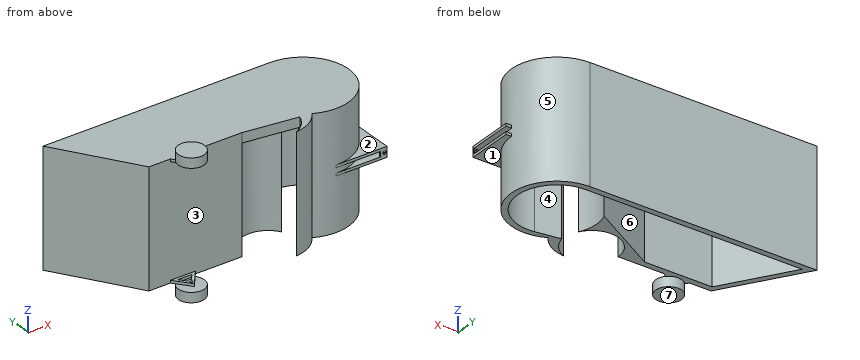
```python
from build123d import *

# Parameters (mm, degrees)
BOSS_EXTRUDE1_DEPTH = 897
SKETCH2_R           = 10.767041916
BOSS_EXTRUDE2_DEPTH = 20
BOSS_EXTRUDE3_START = 20
BOSS_EXTRUDE3_DEPTH = 20
SKETCH4_W           = 50
SKETCH4_H           = 50
SKETCH4_R           = 12.5
BOSS_EXTRUDE4_DEPTH = 10
SKETCH5_R           = 100
BOSS_EXTRUDE5_DEPTH = 75
BOSS_EXTRUDE6_START = -75
BOSS_EXTRUDE6_DEPTH = 75


with BuildPart() as part:
    # Sketch1 → Boss-Extrude1 (new body)
    with BuildSketch(Plane.XY):
        with BuildLine():
            add(Edge.make_bspline(
                [(80.115553735, -191.384207833), (181.903017437, -142.41499007), (210.702960853, -28.558773965)],
                knots=[0, 0, 0, 1, 1, 1], degree=2))
            Line((210.702960853, -28.558773965), (401.206683232, -56.895630445))
            ThreePointArc((401.206683232, -56.895630445), (750.24986995, 222.286833017), (446.080798211, 549.785184001))
            Line((446.080798211, 549.785184001), (-1220.08310634, 549.785184001))
            Line((-1220.08310634, 549.785184001), (-894.475187417, 45))
            Line((-894.475187417, 45), (-374.993230006, 45))
            Line((-374.993230006, 45), (160.769466444, 352.592623287))
            ThreePointArc((160.769466444, 352.592623287), (141.659115875, 226.01181659), (176.177724746, 102.738251846))
            ThreePointArc((176.177724746, 102.738251846), (-53.212296367, 196.881158582), (-203.945431646, 0))
            Line((-203.945431646, 0), (-918.997892597, 0))
            Line((-918.997892597, 0), (-1302.659640419, 594.785184001))
            Line((-1302.659640419, 594.785184001), (446.080798211, 594.785184001))
            ThreePointArc((446.080798211, 594.785184001), (786.541848074, 163.629324532), (288.192746113, -67.578967279))
            add(Edge.make_bspline(
                [(80.115553735, -191.384207833), (212.051449387, -178.806537551), (288.192746113, -67.578967279)],
                knots=[0, 0, 0, 1, 1, 1], degree=2))
        make_face()
    extrude(amount=BOSS_EXTRUDE1_DEPTH)

    # Sketch2 → Boss-Extrude2 (add)
    with BuildSketch(Plane.XY.offset(897)):
        Polygon((-753.618518266, 0), (-561.471662121, 0), (-657.545090194, -121.801839924), align=None)
        with Locations((-657.545090194, -89.507472225)):
            Circle(SKETCH2_R, mode=Mode.SUBTRACT)
        with BuildLine():
            Line((-712.370379676, -20), (-602.719800711, -20))
            Line((-602.719800711, -20), (-641.587482876, -69.276426335))
            ThreePointArc((-641.587482876, -69.276426335), (-657.545090194, -63.740430309), (-673.502697511, -69.276426335))
            Line((-673.502697511, -69.276426335), (-712.370379676, -20))
        make_face(mode=Mode.SUBTRACT)
    boss_extrude2 = extrude(amount=-BOSS_EXTRUDE2_DEPTH)

    # Mirror1: Boss-Extrude2 across plane
    add(boss_extrude2.mirror(Plane.XY.offset(448.5)))

    # Sketch3 → Boss-Extrude3 (add)
    with BuildSketch(Plane.XY.offset(448.5).offset(BOSS_EXTRUDE3_START)):
        with BuildLine():
            Line((796.080798211, -105.214815999), (446.080798211, -105.214815999))
            ThreePointArc((446.080798211, -105.214815999), (693.568171626, -2.702189415), (796.080798211, 244.785184001))
            Line((796.080798211, 244.785184001), (838.444150781, 244.785184001))
            Line((838.444150781, 244.785184001), (838.444150781, -105.214815999))
            Line((838.444150781, -105.214815999), (796.080798211, -105.214815999))
        make_face()
    extrude(amount=BOSS_EXTRUDE3_DEPTH)

    # Mirror2: part across plane


with BuildPart() as part_1:
    add(part.part)
    add(part.part.mirror(Plane.XY.offset(448.5)))

    # Sketch4 → Boss-Extrude4 (add)
    with BuildSketch(Plane.XZ.offset(105.214815999)):
        with Locations((813.444150781, 448.5)):
            Rectangle(SKETCH4_W, SKETCH4_H)
        with Locations((820.168886717, 448.5)):
            Circle(SKETCH4_R, mode=Mode.SUBTRACT)
    extrude(amount=-BOSS_EXTRUDE4_DEPTH)

    # Sketch5 → Boss-Extrude5 (add)
    with BuildSketch(Plane.XY.offset(897)):
        with Locations(Location((-657.545090194, -89.507472225, 0), (0, 0, 139.802215435))):
            Circle(SKETCH5_R)
    extrude(amount=BOSS_EXTRUDE5_DEPTH)

    # Mirror3: part across plane


with BuildPart() as part_2:
    add(part_1.part)
    add(part_1.part.mirror(Plane.XY.offset(448.5)))

    # Sketch6 → Boss-Extrude6 (add)
    with BuildSketch(Plane.XY.offset(897).offset(BOSS_EXTRUDE6_START)):
        with BuildLine():
            Line((-203.945431646, 0), (-561.471662121, 0))
            Line((-561.471662121, 0), (-753.618518266, 0))
            Line((-753.618518266, 0), (-918.997892597, 0))
            Line((-918.997892597, 0), (-1302.659640419, 594.785184001))
            Line((-1302.659640419, 594.785184001), (446.080798211, 594.785184001))
            ThreePointArc((446.080798211, 594.785184001), (786.541848074, 163.629324532), (288.192746113, -67.578967279))
            Line((288.192746113, -67.578967279), (-203.945431646, 0))
        make_face()
    extrude(amount=BOSS_EXTRUDE6_DEPTH)


solid = part_2.part
```
For this review, take the finished solid that the model builds, in its own axes (mm). Face numbers are marked on the shaded views. A direction names the side the tool comes from. Round coordinates to 2 decimals unless told otherwise and drop trailing zeros. Write each loop counter-clockwise with the first axis right and the second up, starting at its lowest first coordinate (ties: lowest second). Pieces come first, ordered by that corner, then holes. Notation, with made-up numbers: (77, 86) -> (118, 86) arc R32 ccw to (118, 112) -> close; hole circle Ø7 at (5, 26.5). An arc over 180 degrees is marked (long way). Use one line per item in the form item = value.
1) Take a section at C-C, the plane x = -58. Write out the cut boundary in (y, z).
Found:
outline = (-20.04, 822) -> (195.52, 822) -> (195.52, 0) -> (226.99, 0) -> (226.99, 822) -> (549.79, 822) -> (549.79, 0) -> (594.79, 0) -> (594.79, 897) -> (-20.04, 897) -> close
2) Take a section at D-D, the plane x = 595. Write out the cut boundary in (y, z).
Found:
outline = (-105.21, 408.5) -> (-71.95, 408.5) -> (-71.95, 0) -> (-21.39, 0) -> (-21.39, 822) -> (510.96, 822) -> (510.96, 0) -> (561.52, 0) -> (561.52, 897) -> (-71.95, 897) -> (-71.95, 488.5) -> (-105.21, 488.5) -> (-105.21, 468.5) -> (-71.95, 468.5) -> (-71.95, 428.5) -> (-105.21, 428.5) -> close
3) To check wall thickness, follow L1, parallel to Y at x = -454.5, z = 484.5; L2, parallel to X at y = 286, z = 786; L3, parallel to X at y = 253, z = 86. State the ranges of each line that lie inside material, in increasing order. Write a range as from..to.
Found:
L1 = 0..45, 549.79..594.79
L2 = -1103.48..-1049.93, 44.78..143.88, 748.28..793.65
L3 = -1082.19..-1028.64, -12.7..141.19, 750.97..795.98
4) Clearance check with flat-ended pins moving along their axes: pin 1 (1.5 mm diameter, centred on x = -101.5, y = 420.5, fed in from +Z); pin 2 (8 mm diameter, centred on y = 271, z = 427.5, fed in from -X); pin 3 (4 mm diameter, centred on x = 563, z = 275, fed in from -Y). State where each tip first meets the part, or that it passes through.
Found:
pin_1 = 897
pin_2 = -1096.38
pin_3 = -85.81
5) Take a section at B-B, the plane y = 492.5. Write out the cut boundary in (x, z), and give its area (3 significant figures).
Found:
outline = (-1236.68, 0) -> (-1183.13, 0) -> (-1183.13, 822) -> (624.02, 822) -> (624.02, 0) -> (693.34, 0) -> (693.34, 897) -> (-1236.68, 897) -> close
area = 246,000 mm2
6) Mouldability with a two-part tool opening along Z and no side actions: class the marked faces 1, 2, 3 and 4 as +Z half, -Z half, draft (parallel to the pull), parting line (faces both ways), or undercut.
Found:
face_1 = -Z half
face_2 = +Z half
face_3 = undercut
face_4 = draft
7) Take a section at A-A, the plane x = -494.5. Write out the cut boundary in (y, z), and give its area (3 significant figures).
Found:
outline = (0, 0) -> (45, 0) -> (45, 822) -> (549.79, 822) -> (549.79, 0) -> (594.79, 0) -> (594.79, 897) -> (0, 897) -> close
area = 119,000 mm2
8) Tool access review of the marked faces 5, 6 and 7: name each direction out of +Z, -Z, +X, -X, +Y, -Y from which nothing blocks a thin tool from reaching the whole face with its end or side.
Found:
face_5 = none
face_6 = -Z
face_7 = -Z, +X, -X, +Y, -Y
